from build123d import *


with BuildPart() as part:
    # Sketch1 → Revolve1 (revolve)
    with BuildSketch(Plane.XY, mode=Mode.PRIVATE) as revolve1_sk:
        with BuildLine():
            Line((20.1625, 108), (20, 103))
            Line((20, 103), (12, 103))
            Line((12, 103), (12, 100))
            Line((12, 100), (-12, 100))
            Line((-12, 100), (-12, 103))
            Line((-12, 103), (-20.1625, 103))
            Line((-20.1625, 103), (-20.1625, 108))
            ThreePointArc((-20.1625, 108), (0, 128.1625), (20.1625, 108))
        make_face()
    revolve(revolve1_sk.sketch.rotate(Axis((88.99, 0, 0), (-1, 0, 0)), 90), axis=Axis((88.99, 0, 0), (-1, 0, 0)))


solid = part.part
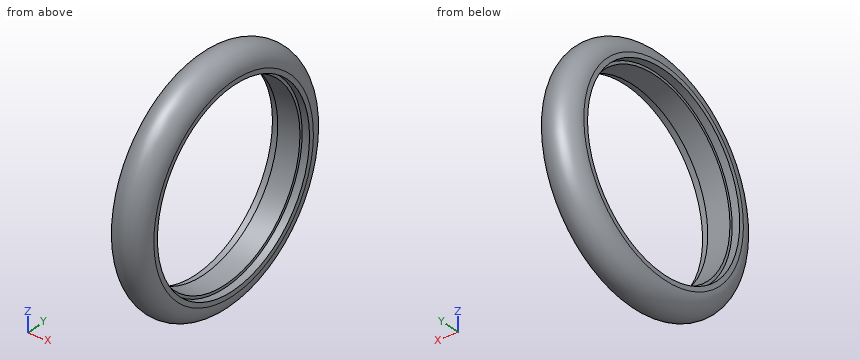
Can you work these out from the model? Positions are in its coordinate system, mm. Give positions to 0.01 mm unless a question says otherwise; leave off trailing zeros. Loops run counter-clockwise (first coordinate to the right, second up) from the corner with the lowest first, then second, coordinate; pieces in that order, holes last. Notation, with made-up numbers: (-27, 59) - (-22, 59) arc R10 cw to (-22, 78) - close; hole circle Ø6 at (66, 21). An arc over 180 degrees is marked (long way). Return JSON: item names as keys, results as strings.
1. I'm going to push flat-ended pins straight in: pin 1 Ø4 at (x, y) = (-14.5, 25.5) entering from +Z; pin 2 Ø6 at (x, z) = (13.5, -95) entering from +Y; pin 3 Ø1.5 at (x, y) = (11.5, -98) entering from -Z. Where does each tip first touch, or does it pass through?
Output values:
{"pin 1": "stops at z = 121.22", "pin 2": "stops at y = 83.13", "pin 3": "stops at z = -78.13"}
2. I want a section at C-C on x = 4. Please give me the cut outline in (y, z).
Output values:
{"outline": "circle Ø255.52 at (0, 0); hole circle Ø200 at (0, 0)"}
3. If I drill on line 1 (X direction, y = -57.5, z = -91.5); line 2 (Y direction, x = -1.5, z = 0); line 3 (Y direction, x = 3.5, z = -48), over which ranges is the centre line in solid material (lowest first)?
Output values:
{"line 1": "x = -20.16 to 20.16", "line 2": "y = -128.11 to -100, 100 to 128.11", "line 3": "y = -118.5 to -87.73, 87.73 to 118.5"}
4. I want a section at A-A on y = 0. Please give me the cut outline in (x, z) (1 decimal).
Output values:
{"outline": "(-20.2, -108) arc R20.2 ccw to (20.2, -108) - (20, -103) - (12, -103) - (12, -100) - (-12, -100) - (-12, -103) - (-20.2, -103) - close; (-20.2, 103) - (-12, 103) - (-12, 100) - (12, 100) - (12, 103) - (20, 103) - (20.2, 108) arc R20.2 ccw to (-20.2, 108) - close"}
